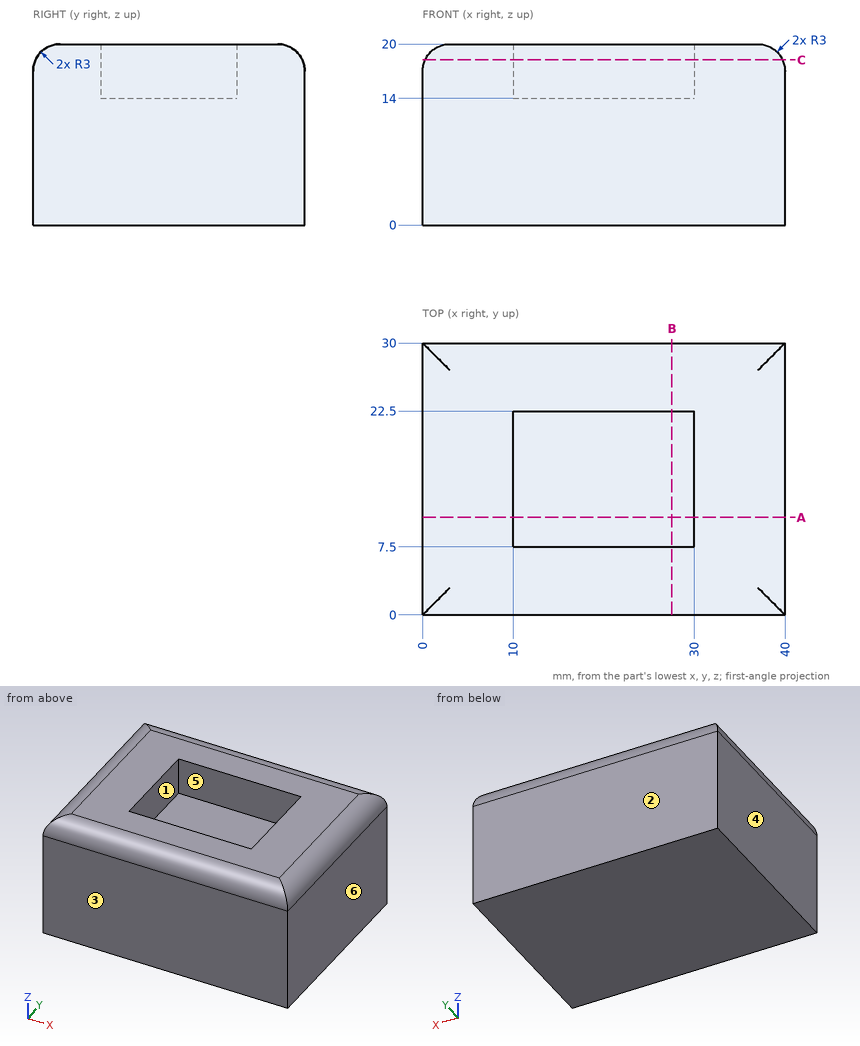
The drawing under review shows one solid part. Ordinate dimensions are in mm from its lowest x, y, z. A direction names the side the tool comes from. Round coordinates to 2 decimals unless told otherwise and drop trailing zeros. Loops run counter-clockwise (first coordinate to the right, second up) from the corner with the lowest first, then second, coordinate; pieces in that order, holes last. Notation, with made-up numbers: (-24, 34.5) -> (10, 34.5) arc R10 cw to (10, 47.5) -> close; hole circle Ø2 at (1.25, -23). An arc over 180 degrees is marked (long way). Answer in a Markdown table with one row per item.
1) Consider section C-C, the plane z = 18.25. Write out the cut boundary in (x, y), plus the area to 3 significant figures.
Taken from the geometry:
| item | result |
|---|---|
| outline | (0.27, 0.27) -> (39.73, 0.27) -> (39.73, 29.73) -> (0.27, 29.73) -> close; hole (10, 7.5) -> (30, 7.5) -> (30, 22.5) -> (10, 22.5) -> close |
| area | 862 mm² |
2) Tool access review of the marked faces 5 and 6: name each direction out of +Z, -Z, +X, -X, +Y, -Y from which nothing blocks a thin tool from reaching the whole face with its end or side.
Taken from the geometry:
| item | result |
|---|---|
| face 5 | +Z |
| face 6 | +Z, -Z, +X, +Y, -Y |
3) Consider section A-A, the plane y = 10.75. Write out the cut boundary in (x, z), plus the area to 3 significant figures.
Taken from the geometry:
| item | result |
|---|---|
| outline | (0, 0) -> (40, 0) -> (40, 17) arc R3 ccw to (37, 20) -> (30, 20) -> (30, 14) -> (10, 14) -> (10, 20) -> (3, 20) arc R3 ccw to (0, 17) -> close |
| area | 676 mm² |
4) Consider section B-B, the plane x = 27.5. Write out the cut boundary in (y, z), plus the area to 3 significant figures.
Taken from the geometry:
| item | result |
|---|---|
| outline | (0, 0) -> (30, 0) -> (30, 17) arc R3 ccw to (27, 20) -> (22.5, 20) -> (22.5, 14) -> (7.5, 14) -> (7.5, 20) -> (3, 20) arc R3 ccw to (0, 17) -> close |
| area | 506 mm² |
5) Wall thickness on line 1 along X through (y, z) = (10.5, 15.5); line 2 along Z through (x, y) = (14.5, 13.75); line 3 along X through (y, z) = (13, 18.75): over which ranges is each line inside the solid? List them lowest first.
Taken from the geometry:
| item | result |
|---|---|
| line 1 | x = 0 to 10, 30 to 40 |
| line 2 | z = 0 to 14 |
| line 3 | x = 0.56 to 10, 30 to 39.44 |
6) For pin 1 Ø7.5 at (x, y) = (20, 18) entering from +Z, flat-tipped, find the tip position at first contact; note if it passes through.
Taken from the geometry:
| item | result |
|---|---|
| pin 1 | stops at z = 14 |
7) Draft analysis for pull direction Y (two halves, no side actions). For the marked faces 1, 2, 3 and 4, state which applies: pulls with the +Y half, pulls with the -Y half, needs draft (parallel to the pull), parting line crosses it, or undercut.
Taken from the geometry:
| item | result |
|---|---|
| face 1 | undercut |
| face 2 | pulls with the +Y half |
| face 3 | pulls with the -Y half |
| face 4 | needs draft |
